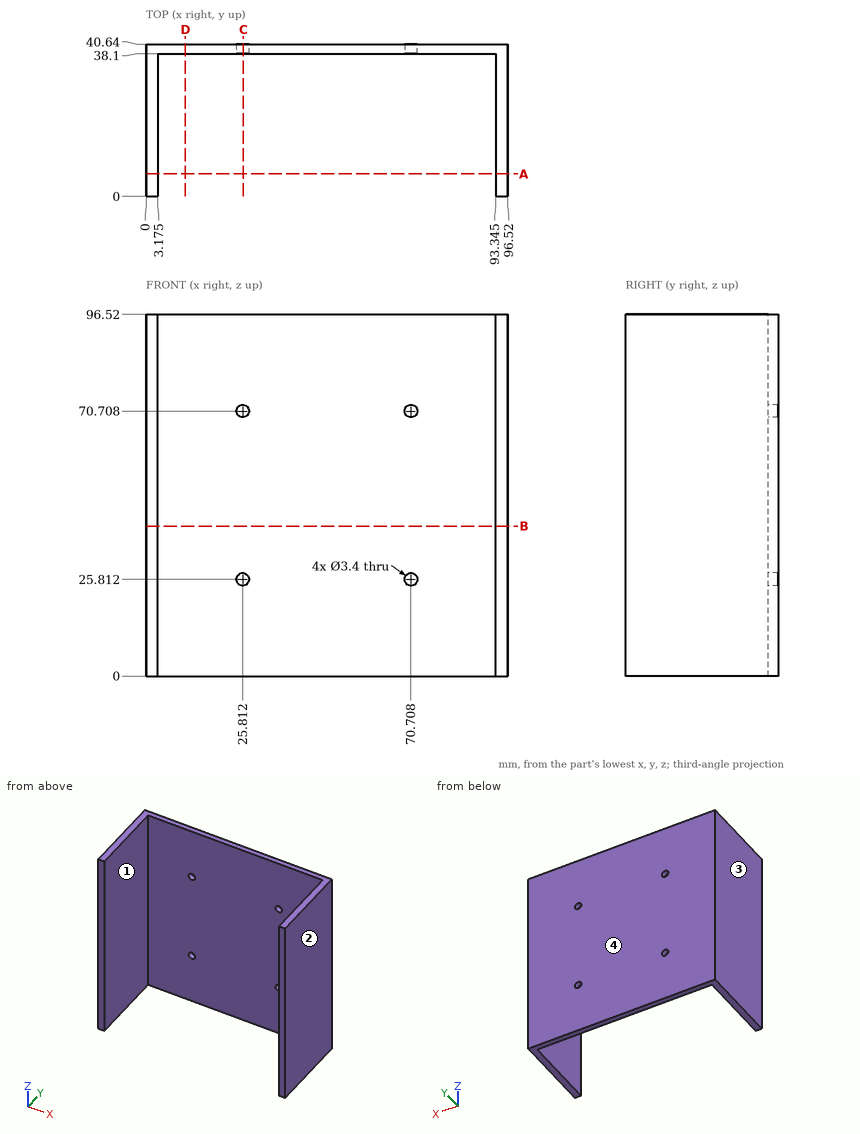
Print and shaded views of the part. All mm, measured from the part's lowest x, y and z. Round coordinates to 2 decimals unless told otherwise and drop trailing zeros. Write each loop counter-clockwise with the first axis right and the second up, starting at its lowest first coordinate (ties: lowest second). Pieces come first, ordered by that corner, then holes. Notation, with made-up numbers: (-21.5, -30.75) - (-5.5, -30.75) arc R15 ccw to (-5.5, -2.75) - close; hole circle Ø5 at (-40, 32.5). An arc over 180 degrees is marked (long way). Use CSV: the item, a comma, the result in double quotes. Start each with the question number.
Item 1: Drill centre lines: L1, parallel to X at y = 29, z = 28.5 (3 decimals); L2, parallel to Y at x = 25, z = 84. Where is each one in solid material? Low to high. Write a range as [from, to].
Item 2: Two-plate mould, pull along X, no slides. Class the marked faces 1, 2, 3 and 4: released by +X, released by -X, zero draft, split by the parting line, or undercut.
Item 3: Pin check, flat tips, straight feed: P1, Ø8, axis at y = 34.5, z = 49.5, coming from the -X side; P2, Ø2, axis at x = 25.81, z = 25.81, coming from the -Y side; P3, Ø10, axis at x = 46, z = 21, coming from the -Y side. Stop position of each tip, or through.
Item 4: Band-saw the part on C-C (x = 26). Write the cut outline in (y, z), and give its area (3 significant figures).
Item 5: Band-saw the part on D-D (x = 10.5). Write the cut outline in (y, z).
Item 6: Band-saw the part on A-A (y = 6). Write the cut outline in (x, z) (3 decimals), and give its area (3 significant figures).
Item 7: Band-saw the part on B-B (z = 40). Write the cut outline in (x, y) (3 decimals).
Checked values:
1,L1,"x = [0, 3.175], [93.345, 96.52]"
1,L2,"y = [38.1, 40.64]"
2,face 1,"undercut"
2,face 2,"released by +X"
2,face 3,"released by -X"
2,face 4,"zero draft"
3,P1,"stops at x = 0"
3,P2,"passes through"
3,P3,"stops at y = 38.1"
4,outline,"(38.1, 0) - (40.64, 0) - (40.64, 24.12) - (38.1, 24.12) - close; (38.1, 27.5) - (40.64, 27.5) - (40.64, 69.02) - (38.1, 69.02) - close; (38.1, 72.4) - (40.64, 72.4) - (40.64, 96.52) - (38.1, 96.52) - close"
4,area,"228 mm²"
5,outline,"(38.1, 0) - (40.64, 0) - (40.64, 96.52) - (38.1, 96.52) - close"
6,outline,"(0, 0) - (3.175, 0) - (3.175, 96.52) - (0, 96.52) - close; (93.345, 0) - (96.52, 0) - (96.52, 96.52) - (93.345, 96.52) - close"
6,area,"613 mm²"
7,outline,"(0, 0) - (3.175, 0) - (3.175, 38.1) - (93.345, 38.1) - (93.345, 0) - (96.52, 0) - (96.52, 40.64) - (0, 40.64) - close"
